Design review of the part built by this model. Coordinates are the model's own, in mm. Face numbers are marked on the shaded views. A direction names the side the tool comes from. Give positions to 0.01 mm unless a question says otherwise; leave off trailing zeros. Loops run counter-clockwise (first coordinate to the right, second up) from the corner with the lowest first, then second, coordinate; pieces in that order, holes last. Notation, with made-up numbers: M -39.5,-34 L -26.5,-34 A23 cw -26.5,-18 Z; hole C 38,84 d5. An arc over 180 degrees is marked long. Use CSV: the item, a comma, the result in double quotes.
from build123d import *

# Parameters (mm, degrees)
RESSALTO_EXTRUS_O1_DEPTH = 10
ESBO_O2_R                = 8.5
RESSALTO_EXTRUS_O2_DEPTH = 70
ESBO_O3_W                = 6
ESBO_O3_H                = 3.485279131
CORTE_EXTRUS_O1_DEPTH    = 40
FILETE1_R                = 2
CHANFRO1_SIZE            = 1


with BuildPart() as part:
    # Esboço1 → Ressalto-extrusão1 (new body)
    with BuildSketch(Plane.XY):
        Polygon((0, 17.320508076), (-15, 8.660254038), (-15, -8.660254038), (0, -17.320508076), (15, -8.660254038), (15, 8.660254038), align=None)
    extrude(amount=-RESSALTO_EXTRUS_O1_DEPTH)

    # Esboço2 → Ressalto-extrusão2 (add)
    with BuildSketch(Plane(origin=(0, 0, -10), x_dir=(-1, 0, 0), z_dir=(0, 0, -1))):
        Circle(ESBO_O2_R)
    extrude(amount=RESSALTO_EXTRUS_O2_DEPTH)

    # Esboço3 → Corte-extrusão1 (cut)
    with BuildSketch(Plane(origin=(0, 0, -80), x_dir=(-1, 0, 0), z_dir=(0, 0, -1))):
        with Locations((0, -7.042639566)):
            Rectangle(ESBO_O3_W, ESBO_O3_H)
    extrude(amount=-CORTE_EXTRUS_O1_DEPTH, mode=Mode.SUBTRACT)

    # Filete1
    filete1_edges = [part.edges().sort_by_distance(p)[0] for p in [
        (-3, -6.62649343, -40),
        (3, -6.62649343, -40),
    ]]
    fillet(filete1_edges, radius=FILETE1_R)

    # Chanfro1
    chanfro1_edges = [part.edges().sort_by_distance(p)[0] for p in [
        (4.834769901, 6.991065727, -80),
    ]]
    chamfer(chanfro1_edges, length=CHANFRO1_SIZE)


solid = part.part
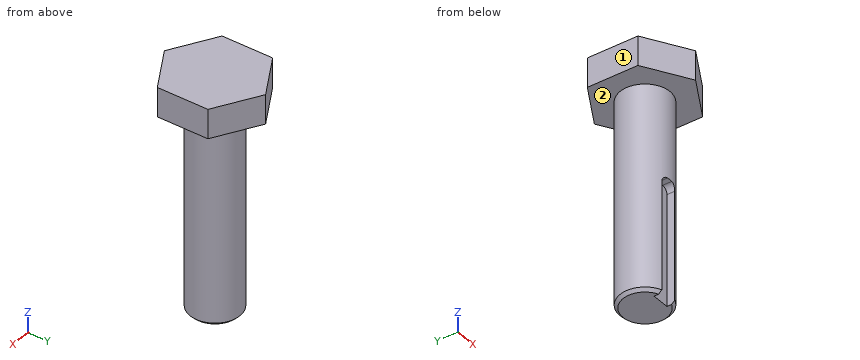
(1) Clearance check with flat-ended pins moving along their axes: P1, Ø2, axis at x = 10, y = -6.5, coming from the -Z side; P2, Ø3, axis at x = 0.5, z = -50.5, coming from the -Y side; P3, Ø6, axis at x = 10.5, z = -46, coming from the +Y side. State where each tip first meets the part, or that it passes through.
A:
P1,"z = -10"
P2,"y = -5.3"
P3,"y = 4"
(2) Wall thickness on line 1 along Z through (x, y) = (2.75, -12.5); line 2 along X through (y, z) = (0, -76); line 3 along X through (y, z) = (-1.5, -23.5): over which ranges is each line inside the solid? List them lowest first. Write a range as [from, to].
A:
line 1,"[-10, 0]"
line 2,"[-8.5, 8.5]"
line 3,"[-8.37, 8.37]"
(3) We need section C-C on z = -63.5. State the section outline as (x, y) points, then the cut area to 3 significant figures.
A:
outline,"M -3,-7.95 L -3,-5.3 L 3,-5.3 L 3,-7.95 A8.5 ccw long Z"
area,"209 mm²"
(4) We need section A-A on y = 0. State the section outline as (x, z) points.
A:
outline,"M -15,-10 L -8.5,-10 L -8.5,-79 L -7.5,-80 L 7.5,-80 L 8.5,-79 L 8.5,-10 L 15,-10 L 15,0 L -15,0 Z"
(5) Machinability: for the marked faces 1 and 2, which of the approach directions +Z, -Z, +X, -X, +Y, -Y give a long, thin tool a straight path to every point of the face, cutting with its end or side? Answer none if there is none.
A:
face 1,"+Z, -Z, -X, +Y, -Y"
face 2,"-Z"
(6) We need section D-D on y = 14.5. State the section outline as (x, z) points.
A:
outline,"M -4.89,-10 L 4.89,-10 L 4.89,0 L -4.89,0 Z"
(7) We need section B-B on z = -26. State the section outline as (x, y) points, then the cut area to 3 significant figures.
A:
outline,"C 0,0 d17"
area,"227 mm²"
